Autodesk Inventor part; units mm, degrees
ref_plane "YZ Plane" through (0, 0, 0) normal (1, 0, 0) x (0, 1, 0)
ref_plane "XZ Plane" through (0, 0, 0) normal (0, 1, 0) x (-1, 0, 0)
ref_plane "XY Plane" through (0, 0, 0) normal (0, 0, 1) x (1, 0, 0)
sketch "Sketch1" plane through (0, 0, 0) normal (0, 0, 1) x (1, 0, 0)
  circle A0 centre (0, -110) radius 125
  circle A1 centre (0, -220) radius 4
  circle A2 centre (110, -110) radius 4
  circle A3 centre (-110, -110) radius 4
  circle A4 centre (0, 0) radius 4
  circle A5 centre (0, -110) radius 125
  circle A6 centre (-7.5, -97.0096) radius 2 construction
  circle A7 centre (-15, -110) radius 2 construction
  circle A8 centre (-7.5, -122.9904) radius 2 construction
  circle A9 centre (7.5, -122.9904) radius 2 construction
  circle A10 centre (15, -110) radius 2 construction
  circle A11 centre (7.5, -97.0096) radius 2 construction
  circle A12 centre (0, -110) radius 29
  dimension "d0" = 58
extrude "Extrusion1" add sketch "Sketch1" along normal blind 5
properties part number "second copper plate" material "Copper"
The listing builds one solid part. Answer for the finished solid, in the listing's coordinates (mm). Round coordinates to 2 decimals unless told otherwise and drop trailing zeros. Loops run counter-clockwise (first coordinate to the right, second up) from the corner with the lowest first, then second, coordinate; pieces in that order, holes last.
Q1. For a pull along Y with two mould halves and no side action, classify faces 1 (the face through (-27.098, 12.028, 2.465)), 2 (the face through (-0.867, 3.905, 2.465)), 3 (the face through (-30, -108, 5)) as released by +Y, released by -Y, zero draft, split by the parting line, or undercut.
Q2. Find the intervals of material crossed by line 1 (Y direction, x = 0, z = 2.6); line 2 (Y direction, x = 110, z = 3.2); line 3 (Y direction, x = -113, z = 2.35), in increasing order.
Q3. Section C-C, the plane y = -97.5 is taken. Determine the outline of the cut face in (x, z), then the cut area to 3 significant figures.
Q4. Section D-D, the plane x = 110 is taken. Determine the outline of the cut face in (y, z), then the cut area to 3 significant figures.
Q5. Section B-B, the plane z = 3.55 is taken. Determine the outline of the cut face in (x, y).
Q6. Given pin 1 Ø1 at (x, z) = (16, 3.5) entering from -Y, flat-ended and moving along its own axis, determine where the tip first touches the part or whether it passes through.
Q7. Section A-A, the plane x = 0 is taken. Determine the outline of the cut face in (y, z), then the cut area to 3 significant figures.
Completed:
1. face 1: split by the parting line
1. face 2: undercut
1. face 3: zero draft
2. line 1: y = -235 to -224, -216 to -139, -81 to -4, 4 to 15
2. line 2: y = -169.37 to -114, -106 to -50.63
2. line 3: y = -163.44 to -112.65, -107.35 to -56.56
3. outline: (-124.37, 0) - (-26.17, 0) - (-26.17, 5) - (-124.37, 5) - close; (26.17, 0) - (124.37, 0) - (124.37, 5) - (26.17, 5) - close
3. area: 982 mm2
4. outline: (-169.37, 0) - (-114, 0) - (-114, 5) - (-169.37, 5) - close; (-106, 0) - (-50.63, 0) - (-50.63, 5) - (-106, 5) - close
4. area: 554 mm2
5. outline: circle Ø250 at (0, -110); hole circle Ø8 at (-110, -110); hole circle Ø58 at (0, -110); hole circle Ø8 at (0, -220); hole circle Ø8 at (0, 0); hole circle Ø8 at (110, -110)
6. pin 1: stops at y = -234.04
7. outline: (-235, 0) - (-224, 0) - (-224, 5) - (-235, 5) - close; (-216, 0) - (-139, 0) - (-139, 5) - (-216, 5) - close; (-81, 0) - (-4, 0) - (-4, 5) - (-81, 5) - close; (4, 0) - (15, 0) - (15, 5) - (4, 5) - close
7. area: 880 mm2
